Verification items for this drawing (mm, ordinates from the low corner). Round coordinates to 2 decimals unless told otherwise and drop trailing zeros. Loops run counter-clockwise (first coordinate to the right, second up) from the corner with the lowest first, then second, coordinate; pieces in that order, holes last. Notation, with made-up numbers: M 88,14 L 104,14 A31 cw 104,41 Z; hole C 20.5,29 d4. An arc over 180 degrees is marked long. One line per item, written item: value.
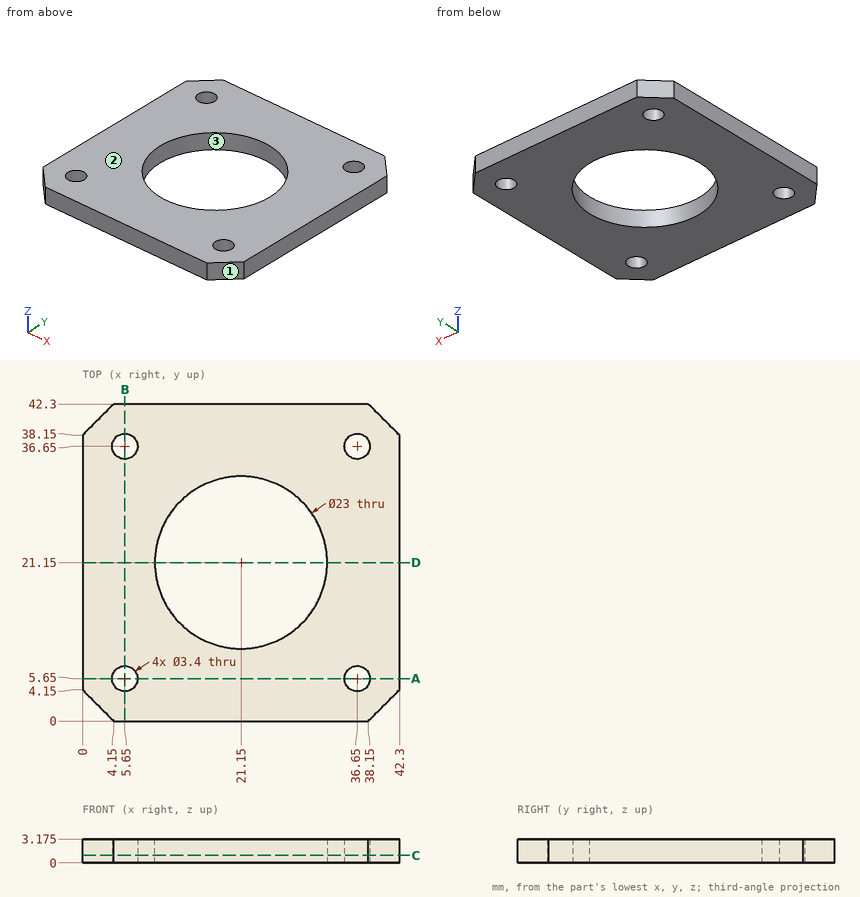
(1) Mould release check, pull along Y, two halves, no side actions. Record for the marked faces 1, 2 and 3: +Y half, -Y half, draft (parallel to the pull), parting line (faces both ways), or undercut.
Completed:
face 1: -Y half
face 2: draft
face 3: undercut
(2) Sectioned sample at A-A on y = 5.65. Enter the section's corners in (x, z) (3 decimals).
Completed:
outline: M 0,0 L 3.95,0 L 3.95,3.175 L 0,3.175 Z; M 7.35,0 L 34.95,0 L 34.95,3.175 L 7.35,3.175 Z; M 38.35,0 L 42.3,0 L 42.3,3.175 L 38.35,3.175 Z
(3) Sectioned sample at C-C on z = 1. Enter the section's corners in (x, y).
Completed:
outline: M 0,4.15 L 4.15,0 L 38.15,0 L 42.3,4.15 L 42.3,38.15 L 38.15,42.3 L 4.15,42.3 L 0,38.15 Z; hole C 5.65,5.65 d3.4; hole C 5.65,36.65 d3.4; hole C 21.15,21.15 d23; hole C 36.65,5.65 d3.4; hole C 36.65,36.65 d3.4
(4) Thickness scan on L1, parallel to Y at x = 5.65, z = 1.45; L2, parallel to Y at x = 36, z = 0.9; L3, parallel to X at y = 30, z = 2.4. Record the ranges inside material, lowest first. Write a range as from..to.
Completed:
L1: y = 0..3.95, 7.35..34.95, 38.35..42.3
L2: y = 0..4.08, 7.22..35.08, 38.22..42.3
L3: x = 0..13.81, 28.49..42.3
(5) Sectioned sample at D-D on y = 21.15. Enter the section's corners in (x, z) (3 decimals).
Completed:
outline: M 0,0 L 9.65,0 L 9.65,3.175 L 0,3.175 Z; M 32.65,0 L 42.3,0 L 42.3,3.175 L 32.65,3.175 Z
